Autodesk Inventor part; units mm, degrees
ref_plane "YZ Plane" through (0, 0, 0) normal (1, 0, 0) x (0, 1, 0)
ref_plane "XZ Plane" through (0, 0, 0) normal (0, 1, 0) x (-1, 0, 0)
ref_plane "XY Plane" through (0, 0, 0) normal (0, 0, 1) x (1, 0, 0)
sketch "Skizze1" plane through (0, 0, 0) normal (0, 0, 1) x (1, 0, 0)
  line L0 (0, 0) -> (14, 0)
  line L1 (0, 2.25) -> (14, 2.25)
  line L2 (14, 2.25) -> (14, 7.25)
  line L3 (14, 7.25) -> (11.5, 7.25)
  line L4 (11.5, 7.25) -> (11.5, 4.25)
  line L5 (11.5, 4.25) -> (2.5, 4.25)
  line L6 (2.5, 4.25) -> (2.5, 7.25)
  line L7 (2.5, 7.25) -> (0, 7.25)
  line L8 (0, 7.25) -> (0, 2.25)
  dimension "d0" = 14
  dimension "d1" = 4.5
  dimension "d2" = 2
  dimension "d3" = 3
  dimension "d4" = 3
  dimension "d5" = 9
revolve "Umdrehung1" add sketch "Skizze1" angle 360 about axis through (0, 0, 0) along (1, 0, 0)
chamfer "Fasen2" distance 1.5 distance2 1 1 edges at (2.5, -7.25, 0) measured on face at (2.5, 6.1798, -0.5783)
chamfer "Fasen3" distance 1 distance2 1.5 1 edges at (11.5, -7.25, 0) measured on face at (13.1667, 7.1561, -1.163)
properties part number "Hülse zum einhaken"
Design review of the part built by this model. Coordinates are the model's own, in mm. A direction names the side the tool comes from. Give positions to 0.01 mm unless a question says otherwise; leave off trailing zeros. Order: outer loops, then holes, each group sorted by start corner. A loop starts at its lowest first (then second) coordinate and runs counter-clockwise, first axis right, second up. Notation, with made-up numbers: (-8.75, 19) -> (41.25, 19) arc R26 ccw to (41.25, 56) -> close; hole circle Ø5 at (5, -30.5). An arc over 180 degrees is marked (long way). Write item = value, one per line. Start each with the question number.
(1) We need section C-C on x = 7.25. Write out the cut boundary in (y, z).
(2) For faces 4 (the face through (2.5, -2, -4)), 5 (the face through (14, 2, 2)), list the 3-axis set-ups (+Z, -Z, +X, -X, +Y, -Y) from which the entire face can be reached by the end or side of a thin tool; tool diameter is ignored.
(3) Mouldability with a two-part tool opening along Z and no side actions: class faces 1 (the face through (11.5, -2, -4)), 2 (the face through (7.1, -0.29, 2.23)), 3 (the face through (6.937, 2.285, -3.584)) as +Z half, -Z half, draft (parallel to the pull), parting line (faces both ways), or undercut.
(4) To check wall thickness, follow line 1 along Z through (x, y) = (6, 0); line 2 along X through (y, z) = (-4.75, -1); line 3 along Z through (x, y) = (7.25, -1). State the ranges of each line that lie inside material, in increasing order.
(5) We need section A-A on z = 0. Write out the cut boundary in (x, y).
(6) For pin 1 (6 mm diameter, centred on x = 8, z = 1.5, fed in from +Y); pin 2 (1 mm diameter, centred on x = 2.5, z = 3.5, fed in from -Y); pin 3 (5 mm diameter, centred on x = 2, y = 3.5, fed in from -Z), all flat-tipped, find the tip position at first contact; note any pin that passes through.
Numbers:
q1.outline = circle Ø8.5 at (0, 0); hole circle Ø4.5 at (0, 0)
q2.face_4 = none
q2.face_5 = +Z, -Z, +X, +Y, -Y
q3.face_1 = draft
q3.face_2 = undercut
q3.face_3 = parting line
q4.line_1 = -4.25 to -2.25, 2.25 to 4.25
q4.line_2 = 0 to 2.5, 11.5 to 14
q4.line_3 = -4.13 to -2.02, 2.02 to 4.13
q5.outline = (0, -7.25) -> (1.5, -7.25) -> (2.5, -5.75) -> (2.5, -4.25) -> (11.5, -4.25) -> (11.5, -5.75) -> (12.5, -7.25) -> (14, -7.25) -> (14, -2.25) -> (0, -2.25) -> close; (0, 2.25) -> (14, 2.25) -> (14, 7.25) -> (12.5, 7.25) -> (11.5, 5.75) -> (11.5, 4.25) -> (2.5, 4.25) -> (2.5, 5.75) -> (1.5, 7.25) -> (0, 7.25) -> close
q6.pin_1 = 4.25
q6.pin_2 = -5.53
q6.pin_3 = -7.17
